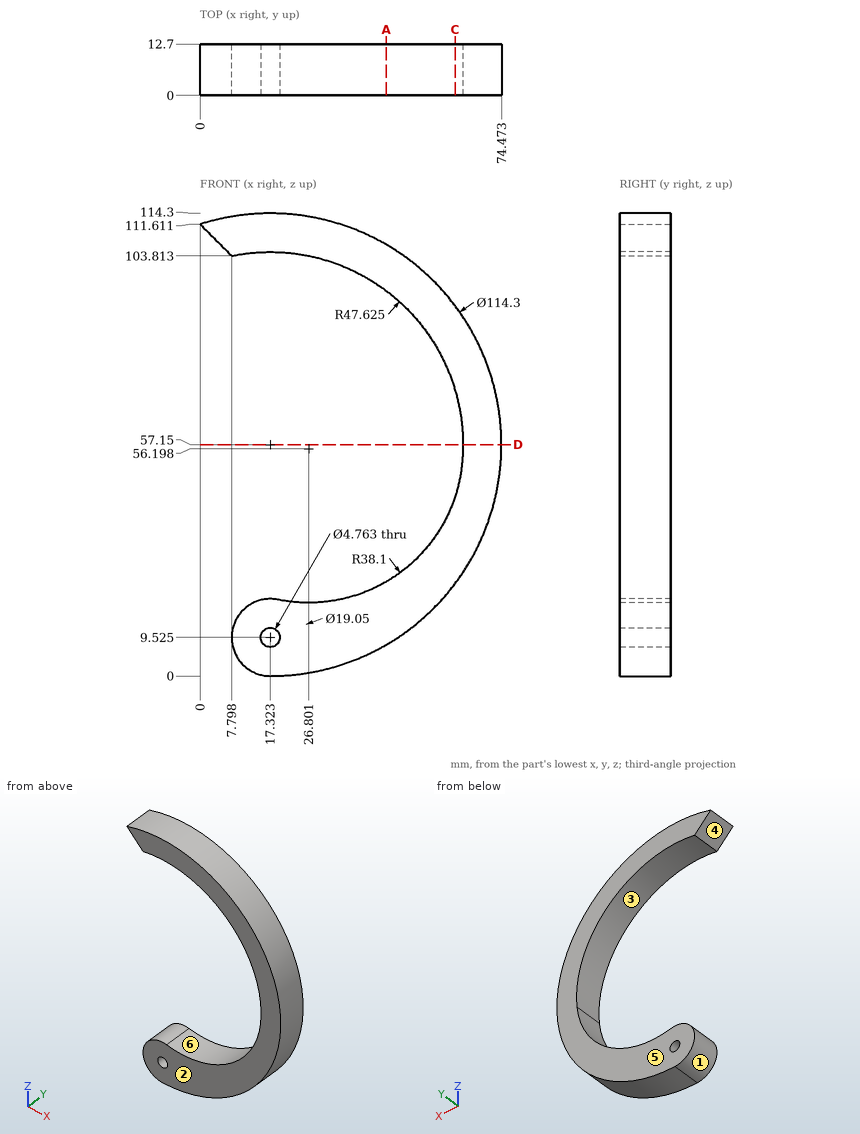
Source: three-view drawing plus pictorial views. Frame: mm from the lowest corner of the part. A direction names the side the tool comes from. Round coordinates to 2 decimals unless told otherwise and drop trailing zeros. Loops run counter-clockwise (first coordinate to the right, second up) from the corner with the lowest first, then second, coordinate; pieces in that order, holes last.
Q1. Ray query, line 1 (Z direction, x = 17, y = 4.25) (1 decimal); line 2 (Z direction, x = 16, y = 0.5) (1 decimal); line 3 (Z direction, x = 27, y = 0.75) (1 decimal). Return the intervals inside material, ascending.
Q2. Access query for the marked faces 5 and 6. Directions: +Z, -Z, +X, -X, +Y, -Y. A direction counts if a zero-diameter tool reaches every point of the face in a straight line with its end or side. Return the directions, or none.
Q3. Mould query, pull axis Z, two halves, no side actions, for the marked faces 1, 2, 3 and 4. Classes: pulls with the +Z half, pulls with the -Z half, needs draft (parallel to the pull), parting line crosses it, or undercut.
Q4. Section C-C, the plane x = 63. Return loops of the section in (y, z), plus the area to 3 significant figures.
Q5. Section A-A, the plane x = 46. Return loops of the section in (y, z) (1 decimal), plus the area to 3 significant figures.
Q6. First-contact query: P1, Ø6, axis at x = 36.5, y = 5.5, coming from the -Z side; P2, Ø5, axis at x = 38.5, y = 1.5, coming from the -Z side; P3, Ø2, axis at x = 8, y = 3.5, coming from the -Z side (1 decimal). Flat tips, straight axial feed; report the tip coordinate or a pass-through.
Q7. Section D-D, the plane z = 57.15. Return loops of the section in (x, y), plus the area to 3 significant figures.
Solutions:
1. line 1: z = 0 to 7.2, 11.9 to 19, 104.8 to 114.3
1. line 2: z = 0.1 to 7.5, 11.5 to 19, 104.8 to 114.3
1. line 3: z = 0.8 to 18.1, 103.8 to 113.5
2. face 5: +Z, -Z, +X, -X, +Y
2. face 6: +Y, -Y
3. face 1: undercut
3. face 2: needs draft
3. face 3: undercut
3. face 4: pulls with the -Z half
4. outline: (0, 22.8) - (12.7, 22.8) - (12.7, 44.31) - (0, 44.31) - close; (0, 70.63) - (12.7, 70.63) - (12.7, 91.5) - (0, 91.5) - close
4. area: 538 mm2
5. outline: (0, 7.7) - (12.7, 7.7) - (12.7, 23.3) - (0, 23.3) - close; (0, 95.2) - (12.7, 95.2) - (12.7, 106.6) - (0, 106.6) - close
5. area: 343 mm2
6. P1: stops at z = 2.34
6. P2: stops at z = 3.14
6. P3: stops at z = 4.9
7. outline: (64.95, 0) - (74.47, 0) - (74.47, 12.7) - (64.95, 12.7) - close
7. area: 121 mm2
